Check sheet for the modelled part. Datum: model origin and axes. Units: mm. A direction names the side the tool comes from. Round coordinates to 2 decimals unless told otherwise and drop trailing zeros. Write each loop counter-clockwise with the first axis right and the second up, starting at its lowest first coordinate (ties: lowest second). Pieces come first, ordered by that corner, then holes. Notation, with made-up numbers: (10, 58.25) - (56, 58.25) arc R22 ccw to (56, 71.25) - close; hole circle Ø10 at (-8.75, 54.5). An arc over 180 degrees is marked (long way). Answer as a JSON object with one key per item and string values. Group by question number.
Item 1: Set-up check for faces 5 (the flat face through (74.447, 13, 160)), 6 (the cylindrical face through (6.421, 12.611, 168.452)), 7 (the flat face through (4.293, 13, 127)), 8 (the flat face through (40, 4, 43.18)): record each of +Z, -Z, +X, -X, +Y, -Y from which the full face is reachable in a straight line by a thin tool's end or side.
Item 2: Sectioned sample at B-B on x = 18.5. Record the boundary of the cut face in (y, z).
Item 3: Sectioned sample at C-C on z = 31. Record the boundary of the cut face in (x, y).
Item 4: Thickness scan on line 1 (Y direction, x = 33, z = 77.5); line 2 (X direction, y = 4.25, z = 73); line 3 (X direction, y = 9, z = 120). Record the ranges inside material, lowest first.
Item 5: Gauge pin test, flat ends, axial feed: P1, Ø6.5, axis at y = 13, z = 128, coming from the -X side; P2, Ø4, axis at x = 41, z = 74, coming from the +Y side; P3, Ø6.5, axis at y = 13, z = 125.5, coming from the +X side. Record the tip position at first contact, or that the pin passes through.
Item 6: Sectioned sample at A-A on z = 139.5. Record the boundary of the cut face in (x, y), plus the area to 3 significant figures.
Item 7: Release check for a two-part mould opening along Z. For faces 1 (the cylindrical face through (72.319, 12.611, 118.568)), 2 (the flat face through (40, 4, 5.08)), 3 (the flat face through (70.282, 13, 160)), 4 (the cylindrical face through (72.41, 12.611, 135.432)) record: pulls with the +Z half, pulls with the -Z half, needs draft (parallel to the pull), parting line crosses it, or undercut.
```python
from build123d import *

# Parameters (mm, degrees)
SKETCH1_W            = 78.74
SKETCH1_H            = 203.2
BOSS_EXTRUDE1_DEPTH  = 6.35
BOSS_EXTRUDE2_DEPTH  = 12.7
LPATTERN2_COUNT      = 2
LPATTERN2_PITCH      = 65.9892
LPATTERN2_COUNT_DIR2 = 2
LPATTERN2_PITCH_DIR2 = 33.02
SKETCH3_W            = 38.1
SKETCH3_H            = 3.81
CUT_EXTRUDE1_DEPTH   = 219.753583056
FILLET1_R            = 2.54


with BuildPart() as part:
    # Sketch1 → Boss-Extrude1 (new body)
    with BuildSketch(Plane(origin=(0, 0, 0), x_dir=(1, 0, 0), z_dir=(0, 1, 0))):
        with Locations((39.37, -101.6)):
            Rectangle(SKETCH1_W, SKETCH1_H)
    extrude(amount=BOSS_EXTRUDE1_DEPTH)

    # Sketch2 → Boss-Extrude2 (add)
    with BuildSketch(Plane(origin=(0, 6.35, 0), x_dir=(1, 0, 0), z_dir=(0, 1, 0))):
        with BuildLine():
            Line((4.2926, -133.35), (4.2926, -120.65))
            ThreePointArc((4.2926, -120.65), (6.3754, -118.5672), (8.4582, -120.65))
            Line((8.4582, -120.65), (8.4582, -133.35))
            ThreePointArc((8.4582, -133.35), (6.3754, -135.4328), (4.2926, -133.35))
        make_face()
    boss_extrude2 = extrude(amount=BOSS_EXTRUDE2_DEPTH)

    # LPattern2: Boss-Extrude2 2 × 2
    with Locations(*[(i * LPATTERN2_PITCH, 0, j * LPATTERN2_PITCH_DIR2) for i in range(LPATTERN2_COUNT) for j in range(LPATTERN2_COUNT_DIR2) if (i, j) != (0, 0)]):
        add(boss_extrude2)

    # Sketch3 → Cut-Extrude1 (cut, through all)
    with BuildSketch(Plane(origin=(78.74, 0, 0), x_dir=(0, 0, -1), z_dir=(1, 0, 0))):
        with Locations((-24.13, 4.445)):
            Rectangle(SKETCH3_W, SKETCH3_H)
    extrude(amount=-CUT_EXTRUDE1_DEPTH, mode=Mode.SUBTRACT)

    # Fillet1
    fillet1_edges = [part.edges().sort_by_distance(p)[0] for p in [
        (78.74, 6.35, 123.19),
        (39.37, 6.35, 0),
        (0, 6.35, 2.54),
        (78.74, 6.35, 2.54),
        (0, 6.35, 123.19),
        (0, 3.175, 0),
        (78.74, 3.175, 0),
        (78.74, 3.175, 203.2),
        (0, 3.175, 203.2),
        (39.37, 6.35, 203.2),
    ]]
    fillet(fillet1_edges, radius=FILLET1_R)


solid = part.part
```
Completed:
{
 "1": {"face 5": "+Z, -Z, +X, +Y", "face 6": "+Z, +Y", "face 7": "+Z, -Z, -X, +Y", "face 8": "+X, -X, +Y"},
 "2": {"outline": "(0, 0) - (3.81, 0) arc R2.54 ccw to (6.35, 2.54) - (6.35, 5.08) - (2.54, 5.08) - (2.54, 43.18) - (6.35, 43.18) - (6.35, 200.66) arc R2.54 ccw to (3.81, 203.2) - (0, 203.2) - close"},
 "3": {"outline": "(0, 0) - (78.74, 0) - (78.74, 2.54) - (0, 2.54) - close"},
 "4": {"line 1": "0 to 6.35", "line 2": "0.04 to 78.7", "line 3": "4.4 to 8.35, 70.39 to 74.34"},
 "5": {"P1": "x = 4.29", "P2": "y = 6.35", "P3": "x = 74.45"},
 "6": {"outline": "(0, 0) - (78.74, 0) - (78.74, 3.81) arc R2.54 ccw to (76.2, 6.35) - (2.54, 6.35) arc R2.54 ccw to (0, 3.81) - close", "area": "497 mm²"},
 "7": {"face 1": "pulls with the -Z half", "face 2": "undercut", "face 3": "needs draft", "face 4": "undercut"}
}
